Autodesk Inventor part; units mm, degrees
ref_plane "YZ Plane" through (0, 0, 0) normal (1, 0, 0) x (0, 1, 0)
ref_plane "XZ Plane" through (0, 0, 0) normal (0, 1, 0) x (-1, 0, 0)
ref_plane "XY Plane" through (0, 0, 0) normal (0, 0, 1) x (1, 0, 0)
sketch "Sketch1" plane through (0, 0, 0) normal (0, 0, 1) x (1, 0, 0)
  line L0 (20.5, 0) -> (20.5, 8)
  line L1 (20.5, 8) -> (0, 8)
  line L2 (0, 8) -> (0, 0)
  circle A0 centre (3, 2.5) radius 1.25
  circle A1 centre (17.5, 2.5) radius 1.25
  line L3 (4.75, 0) -> (15.75, 0)
  line L4 (15.75, 0) -> (15.75, 6)
  line L5 (15.75, 6) -> (4.75, 6)
  line L6 (4.75, 6) -> (4.75, 0)
  line L7 (0, 0) -> (4.75, 0)
  line L8 (15.75, 0) -> (20.5, 0)
  dimension "d0" = 2.5
  dimension "d1" = 2.5
  dimension "d2" = 14.5
  dimension "d7" = 3
  dimension "d8" = 3
  dimension "d9" = 11
extrude "Extrusion1" add sketch "Sketch1" along normal blind 3 contours L8 L4 L5 L6 L7 L2 L1 L0
extrude "Extrusion2" add sketch "Sketch1" along normal blind 1.5 contours L3 L6 L5 L4
chamfer "Chamfer1" distance 4 angle 45 2 edges at (0, 8, 1.5) (20.5, 8, 1.5)
chamfer "Chamfer2" distance 1.5 angle 45 2 edges at (1.75, 2.5, 0) (16.25, 2.5, 0)
properties part number "switchholder"
Model file for the job. Use its own axes, mm. A direction names the side the tool comes from. Round coordinates to 2 decimals unless told otherwise and drop trailing zeros. Loops run counter-clockwise (first coordinate to the right, second up) from the corner with the lowest first, then second, coordinate; pieces in that order, holes last. Notation, with made-up numbers: M 11.25,14.25 L 32.25,14.25 A36 ccw 32.25,51.25 Z; hole C -15,-12.75 d1. An arc over 180 degrees is marked long. One line per question, with ' | ' between items.
1) Band-saw the part on C-C (z = 1.9). Give the cut face in (x, y), then the cut area to 3 significant figures.
Solved:
outline: M 0,0 L 4.75,0 L 4.75,6 L 15.75,6 L 15.75,0 L 20.5,0 L 20.5,4 L 16.5,8 L 4,8 L 0,4 Z; hole C 3,2.5 d2.5; hole C 17.5,2.5 d2.5 | area: 72.2 mm²
2) Flat gauge pins, fed straight in: pin 1 (1.5 mm diameter, centred on x = 4, y = 2, fed in from -Z); pin 2 (1 mm diameter, centred on y = 6.5, z = 1, fed in from +X); pin 3 (3 mm diameter, centred on x = 11.5, y = 2, fed in from +Z); pin 4 (2 mm diameter, centred on x = 17.5, y = 2.5, fed in from +Z). Where does each tip first touch, or does it go through?
Solved:
pin 1: stops at z = 0.88 | pin 2: stops at x = 18.5 | pin 3: stops at z = 1.5 | pin 4: passes through
3) Band-saw the part on B-B (x = 3). Give the cut face in (y, z), then the cut area to 3 significant figures.
Solved:
outline: M 0,0.25 L 1.25,1.5 L 1.25,3 L 0,3 Z; M 3.75,1.5 L 5.25,0 L 7,0 L 7,3 L 3.75,3 Z | area: 11.3 mm²
4) 3-axis set-ups, long thin cutter, end or side, ignore diameter. For faces 5 (the cylindrical face through (4.19, 2.12, 2.24)), 6 (the flat face through (10, 6, 2)): which of +Z, -Z, +X, -X, +Y, -Y reach the whole face in a straight line?
Solved:
face 5: +Z, -Z | face 6: +Z, -Y
5) Drill centre lines: line 1 along X through (y, z) = (3, 2.65); line 2 along X through (y, z) = (5.75, 2.4); line 3 along Z through (x, y) = (9, 2.5). Where is each one in solid material? Low to high.
Solved:
line 1: x = 0 to 1.85, 4.15 to 4.75, 15.75 to 16.35, 18.65 to 20.5 | line 2: x = 1.75 to 4.75, 15.75 to 18.75 | line 3: z = 0 to 1.5
6) Band-saw the part on A-A (y = 2.5). Give the cut face in (x, z).
Solved:
outline: M 0,0 L 0.25,0 L 1.75,1.5 L 1.75,3 L 0,3 Z; M 4.25,1.5 L 5.75,0 L 14.75,0 L 16.25,1.5 L 16.25,3 L 15.75,3 L 15.75,1.5 L 4.75,1.5 L 4.75,3 L 4.25,3 Z; M 18.75,1.5 L 20.25,0 L 20.5,0 L 20.5,3 L 18.75,3 Z
7) Mould opens along X. For faces 1 (the flat face through (15.75, 3, 2)), 2 (the flat face through (10, 7, 3)), 3 (the flat face through (0, 2, 1)), 4 (the flat face through (18.5, 6, 1.5)) say: +X half, -X half, draft (parallel to the pull), parting line (faces both ways), or undercut.
Solved:
face 1: undercut | face 2: draft | face 3: -X half | face 4: +X half
8) Band-saw the part on D-D (y = 5.75). Give the cut face in (x, z), then the cut area to 3 significant figures.
Solved:
outline: M 1.75,0 L 18.75,0 L 18.75,3 L 15.75,3 L 15.75,1.5 L 4.75,1.5 L 4.75,3 L 1.75,3 Z | area: 34.5 mm²
